Could you check a few things on this drawing? It's one solid part, dimensions in mm from its lowest x, y, z. A direction names the side the tool comes from. Coordinates: 2 decimals unless noted, no trailing zeros. Order: outer loops, then holes, each group sorted by start corner. A loop starts at its lowest first (then second) coordinate and runs counter-clockwise, first axis right, second up. Notation, with made-up numbers: (-12.75, -25) -> (14.25, -25) arc R25 cw to (14.25, -3) -> close; hole circle Ø3 at (-19.5, 43). An arc over 180 degrees is marked (long way). Use a Markdown table: item, result. Add a question column.
1. Suppose I cut it at C-C, the plane y = 4.75. List the corners of the cut face in (x, z) for me, then the cut area to 3 significant figures.
2. If I drill on line 1 along Z through (x, y) = (1.5, 1.75); line 2 along Y through (x, z) = (1.5, 5.25); line 3 along X through (y, z) = (5.15, 7.5), over which ranges is the centre line in solid material (lowest first)? Write a range as from..to.
3. We'd pull the mould along Z, two halves only. Please class the marked faces 1, 2 and 3: pulls with the +Z half, pulls with the -Z half, needs draft (parallel to the pull), parting line crosses it, or undercut.
4. Suppose I cut it at A-A, the plane x = 7.5. List the corners of the cut face in (y, z) for me, then the cut area to 3 significant figures.
5. For pin 1 Ø3 at (x, z) = (8, 6.5) entering from +Y; pin 2 Ø1.5 at (x, y) = (7, 1) entering from -Z; pin 3 Ø1.5 at (y, z) = (5.5, 6) entering from +X; pin 4 Ø1 at (x, y) = (10, 0.5) entering from +Z, each with a flat end and sliding along its axis, tell me the tip position at first contact or that it passes through.
6. Suppose I cut it at D-D, the plane x = 5.25. List the corners of the cut face in (y, z) for me, then the cut area to 3 significant figures.
7. For the marked faces 4 and 5, which set-ups out of +Z, -Z, +X, -X, +Y, -Y let a thin tool reach every point of the face, with its end or its side?
8. Suppose I cut it at B-B, the plane z = 7.5. List the corners of the cut face in (x, y) for me.
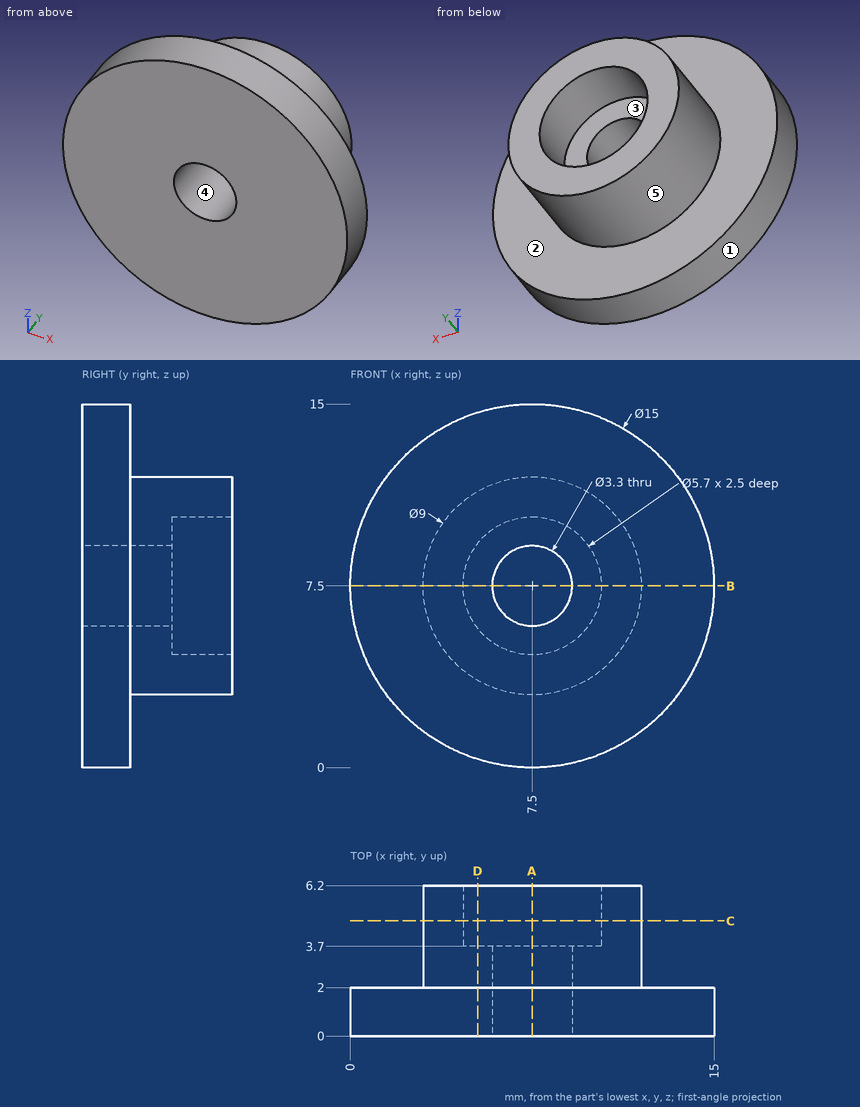
Worked out:
| question | item | result |
|---|---|---|
| 1 | outline | circle Ø9 at (7.5, 7.5); hole circle Ø5.7 at (7.5, 7.5) |
| 1 | area | 38.1 mm² |
| 2 | line 1 | z = 3..12 |
| 2 | line 2 | y = 0..2 |
| 2 | line 3 | x = 3..4.65, 10.35..12 |
| 3 | face 1 | parting line crosses it |
| 3 | face 2 | needs draft |
| 3 | face 3 | undercut |
| 4 | outline | (0, 0) -> (2, 0) -> (2, 3) -> (6.2, 3) -> (6.2, 4.65) -> (3.7, 4.65) -> (3.7, 5.85) -> (0, 5.85) -> close; (0, 9.15) -> (3.7, 9.15) -> (3.7, 10.35) -> (6.2, 10.35) -> (6.2, 12) -> (2, 12) -> (2, 15) -> (0, 15) -> close |
| 4 | area | 41.3 mm² |
| 5 | pin 1 | stops at y = 3.7 |
| 5 | pin 2 | stops at z = 0 |
| 5 | pin 3 | stops at x = 11.94 |
| 5 | pin 4 | stops at z = 14.73 |
| 6 | outline | (0, 0.35) -> (2, 0.35) -> (2, 3.6) -> (6.2, 3.6) -> (6.2, 5.75) -> (3.7, 5.75) -> (3.7, 9.25) -> (6.2, 9.25) -> (6.2, 11.4) -> (2, 11.4) -> (2, 14.65) -> (0, 14.65) -> close |
| 6 | area | 52.6 mm² |
| 7 | face 4 | +Y, -Y |
| 7 | face 5 | +Y |
| 8 | outline | (0, 0) -> (5.85, 0) -> (5.85, 3.7) -> (4.65, 3.7) -> (4.65, 6.2) -> (3, 6.2) -> (3, 2) -> (0, 2) -> close; (9.15, 0) -> (15, 0) -> (15, 2) -> (12, 2) -> (12, 6.2) -> (10.35, 6.2) -> (10.35, 3.7) -> (9.15, 3.7) -> close |
